The model under review builds one solid part; all positions refer to its coordinate system, in mm. Coordinates: 2 decimals unless noted, no trailing zeros. Write each loop counter-clockwise with the first axis right and the second up, starting at its lowest first coordinate (ties: lowest second). Pieces come first, ordered by that corner, then holes. Notation, with made-up numbers: (-37.75, 19) - (-6.75, 19) arc R13 ccw to (-6.75, 41) - close; hole circle Ø5 at (-35.5, -14). An arc over 180 degrees is marked (long way). Put each result on its own line as item: value. Start each with the question number.
Item 1: Consider section A-A on y = 5. Give the boundary of the cut face in (x, z), then the cut area to 3 significant figures.
Item 2: To check wall thickness, follow L1, parallel to Y at x = -11, z = 1.6; L2, parallel to X at y = 16.5, z = 1.25; L3, parallel to X at y = 39, z = 0.5. State the ranges of each line that lie inside material, in increasing order. Write a range as [from, to].
Item 3: Consider section B-B on x = -71. Give the boundary of the cut face in (y, z).
Item 4: Consider section D-D on x = -11. Give the boundary of the cut face in (y, z).
Item 5: Consider section C-C on y = 30. Give the boundary of the cut face in (x, z).
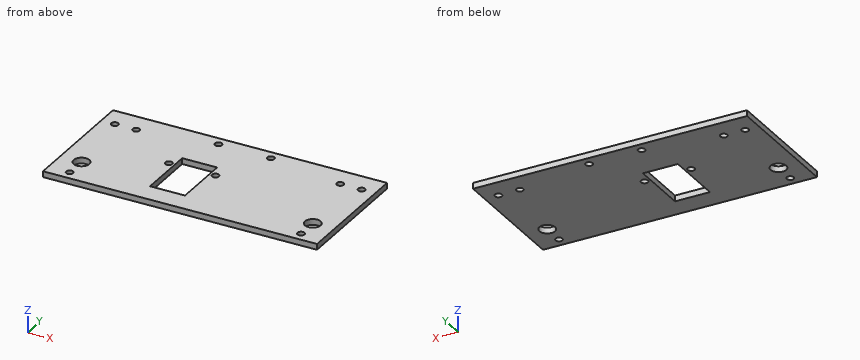
```python
from build123d import *

# Parameters (mm, degrees)
SKETCH_W   = 141
SKETCH_H   = 65.3
SKETCH_R   = 4.05
SKETCH_R_2 = 1.8
SKETCH_W_2 = 18
SKETCH_H_2 = 30
PAD_DEPTH  = 3


with BuildPart() as part:
    # Sketch → Pad (new body)
    with BuildSketch(Plane.XY):
        with Locations((-70.5, 32.65)):
            Rectangle(SKETCH_W, SKETCH_H)
        with Locations((-130, 16)):
            Circle(SKETCH_R, mode=Mode.SUBTRACT)
        with Locations((-11, 16)):
            Circle(SKETCH_R, mode=Mode.SUBTRACT)
        with Locations((-134, 54.3)):
            Circle(SKETCH_R_2, mode=Mode.SUBTRACT)
        with Locations((-123, 54.3)):
            Circle(SKETCH_R_2, mode=Mode.SUBTRACT)
        with Locations((-18, 54.3)):
            Circle(SKETCH_R_2, mode=Mode.SUBTRACT)
        with Locations((-7, 54.3)):
            Circle(SKETCH_R_2, mode=Mode.SUBTRACT)
        with Locations((-84, 60.3)):
            Circle(SKETCH_R_2, mode=Mode.SUBTRACT)
        with Locations((-57, 60.3)):
            Circle(SKETCH_R_2, mode=Mode.SUBTRACT)
        with Locations((-95, 34)):
            Circle(SKETCH_R_2, mode=Mode.SUBTRACT)
        with Locations((-71, 34)):
            Circle(SKETCH_R_2, mode=Mode.SUBTRACT)
        with Locations((-130, 5)):
            Circle(SKETCH_R_2, mode=Mode.SUBTRACT)
        with Locations((-11, 5)):
            Circle(SKETCH_R_2, mode=Mode.SUBTRACT)
        with Locations((-83, 26)):
            Rectangle(SKETCH_W_2, SKETCH_H_2, mode=Mode.SUBTRACT)
    extrude(amount=PAD_DEPTH)


solid = part.part
```
Report:
1. outline: (-141, 0) - (-131.8, 0) - (-131.8, 3) - (-141, 3) - close; (-128.2, 0) - (-12.8, 0) - (-12.8, 3) - (-128.2, 3) - close; (-9.2, 0) - (0, 0) - (0, 3) - (-9.2, 3) - close
1. area: 401 mm²
2. L1: [0, 3.2], [6.8, 11.95], [20.05, 65.3]
2. L2: [-141, -134.02], [-125.98, -92], [-74, -15.02], [-6.98, 0]
2. L3: [-141, -92], [-74, 0]
3. outline: (0, 0) - (32.2, 0) - (32.2, 3) - (0, 3) - close; (35.8, 0) - (65.3, 0) - (65.3, 3) - (35.8, 3) - close
4. outline: (0, 0) - (3.2, 0) - (3.2, 3) - (0, 3) - close; (6.8, 0) - (11.95, 0) - (11.95, 3) - (6.8, 3) - close; (20.05, 0) - (65.3, 0) - (65.3, 3) - (20.05, 3) - close
5. outline: (-141, 0) - (-92, 0) - (-92, 3) - (-141, 3) - close; (-74, 0) - (0, 0) - (0, 3) - (-74, 3) - close
